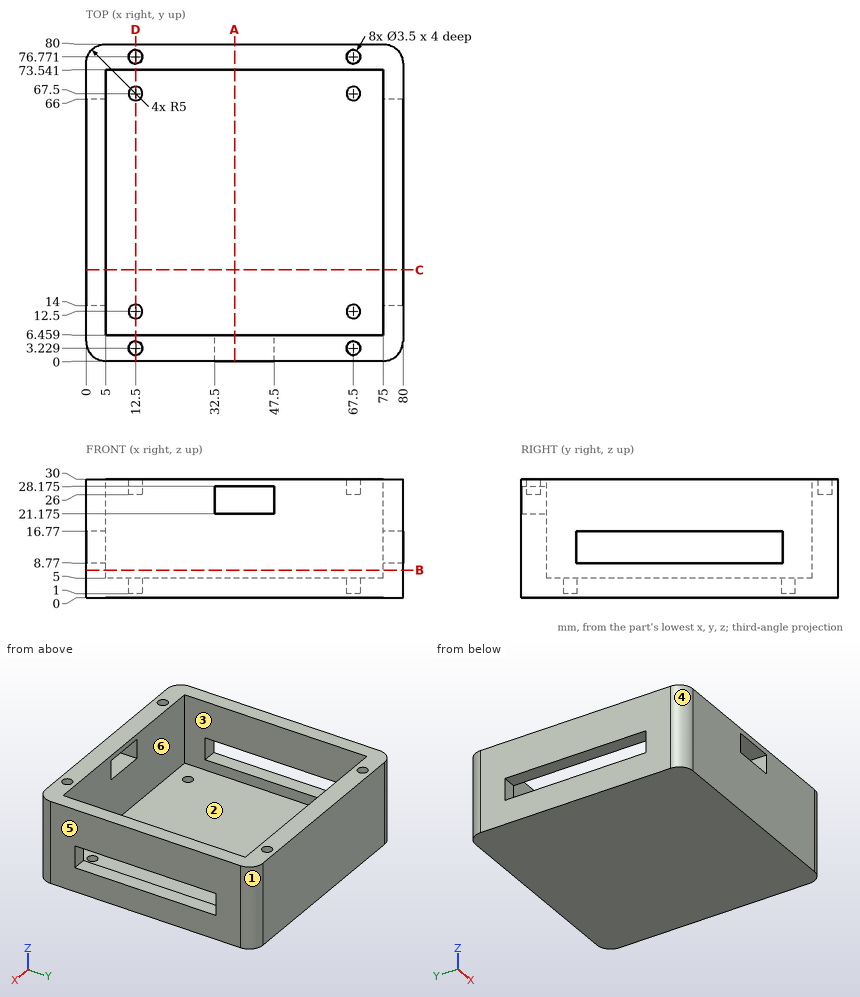
Part print with two shaded views. Sizes in mm from the minimum x, y, z corner. A direction names the side the tool comes from. Coordinates: 2 decimals unless noted, no trailing zeros. Loops run counter-clockwise (first coordinate to the right, second up) from the corner with the lowest first, then second, coordinate; pieces in that order, holes last. Notation, with made-up numbers: (54, 80.25) - (95, 80.25) arc R30 ccw to (95, 118.25) - close; hole circle Ø5 at (54, 5.25). An arc over 180 degrees is marked (long way). Write each question's results on one line, items separated by ' | '. Start each with the question number.
Q1. Which spindle directions (+Z, -Z, +X, -X, +Y, -Y) get a long thin tool onto all of the face, cutting with end or side? Do the marked faces 1 and 2. Say none if no direction does.
Q2. Slice it at D-D on x = 12.5. Give the cut face in (y, z).
Q3. Slice it at B-B on z = 7. Give the cut face in (x, y), and give its area (3 significant figures).
Q4. Slice it at C-C on y = 23. Give the cut face in (x, z).
Q5. Slice it at A-A on x = 37.5. Give the cut face in (y, z) (1 decimal), and give its area (3 significant figures).
Q6. Probe line 1 along Y through (x, z) = (12.5, 3.4); line 2 along Y through (x, z) = (12.5, 28.3). List the from-to ranges inside material, lowest first.
Q7. Two-plate mould, pull along Y, no slides. Class the marked faces 3, 4, 5 and 6: +Y half, -Y half, draft (parallel to the pull), parting line (faces both ways), or undercut.
Q8. Drop flat-ended pins along their axis: pin 1 Ø5 at (x, y) = (38.5, 4.5) entering from -Z; pin 2 Ø3 at (x, y) = (67.5, 76.77) entering from +Z; pin 3 Ø4 at (x, z) = (78, 13) entering from +Y; pin 4 Ø3 at (x, y) = (15.5, 43) entering from +Z. Give the stop position or say it passes through.
Answer:
1) face 1: +Z, -Z, +X, +Y | face 2: +Z
2) outline: (0, 0) - (80, 0) - (80, 30) - (78.52, 30) - (78.52, 26) - (75.02, 26) - (75.02, 30) - (73.54, 30) - (73.54, 5) - (69.25, 5) - (69.25, 1) - (65.75, 1) - (65.75, 5) - (14.25, 5) - (14.25, 1) - (10.75, 1) - (10.75, 5) - (6.46, 5) - (6.46, 30) - (4.98, 30) - (4.98, 26) - (1.48, 26) - (1.48, 30) - (0, 30) - close
3) outline: (0, 5) arc R5 ccw to (5, 0) - (75, 0) arc R5 ccw to (80, 5) - (80, 75) arc R5 ccw to (75, 80) - (5, 80) arc R5 ccw to (0, 75) - close; hole (5, 6.46) - (75, 6.46) - (75, 73.54) - (5, 73.54) - close | area: 1,680 mm2
4) outline: (0, 0) - (80, 0) - (80, 8.77) - (75, 8.77) - (75, 5) - (5, 5) - (5, 8.77) - (0, 8.77) - close; (0, 16.77) - (5, 16.77) - (5, 30) - (0, 30) - close; (75, 16.77) - (80, 16.77) - (80, 30) - (75, 30) - close
5) outline: (0, 0) - (80, 0) - (80, 30) - (73.5, 30) - (73.5, 5) - (6.5, 5) - (6.5, 21.2) - (0, 21.2) - close; (0, 28.2) - (6.5, 28.2) - (6.5, 30) - (0, 30) - close | area: 678 mm2
6) line 1: y = 0 to 10.75, 14.25 to 65.75, 69.25 to 80 | line 2: y = 0 to 1.48, 4.98 to 6.46, 73.54 to 75.02, 78.52 to 80
7) face 3: undercut | face 4: -Y half | face 5: draft | face 6: undercut
8) pin 1: stops at z = 0 | pin 2: stops at z = 26 | pin 3: stops at y = 79.9 | pin 4: stops at z = 5
